For this review, take the finished solid that the model builds, in its own axes (mm). Face numbers are marked on the shaded views. A direction names the side the tool comes from. Give positions to 0.01 mm unless a question says otherwise; leave off trailing zeros. Write each loop counter-clockwise with the first axis right and the second up, starting at its lowest first coordinate (ties: lowest second). Pieces come first, ordered by that corner, then holes. Notation, with made-up numbers: (-19, 18) -> (16, 18) arc R34 ccw to (16, 48) -> close; hole circle Ø7 at (-17.75, 16.5). An arc over 180 degrees is marked (long way). Write item = value, one per line.
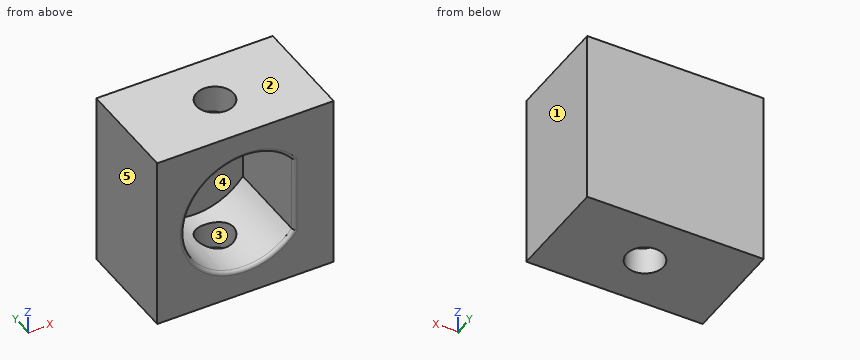
```python
from build123d import *

# Parameters (mm, degrees)
F0_W     = 50
F0_H     = 50
F1_DEPTH = 30
F3_R     = 1
F4_W     = 50
F4_H     = 50
F5_DEPTH = 5
F6_D     = 10.5


with BuildPart() as f1:
    # F0 (on Front) → F1 (new body)
    with BuildSketch(Plane.XZ):
        Rectangle(F0_W, F0_H)
        with BuildLine():
            ThreePointArc((13.65, -10.8710625056), (-17.45, 0), (13.65, 10.8710625056))
            Line((13.65, 10.8710625056), (13.65, -10.8710625056))
        make_face(mode=Mode.SUBTRACT)
    extrude(amount=F1_DEPTH)

    # F3
    f3_edges = [f1.edges().sort_by_distance(p)[0] for p in [
        (13.65, -30, 0),
        (-17.45, -30, 0),
    ]]
    fillet(f3_edges, radius=F3_R)

    # F4 (on face) → F5 (join)
    with BuildSketch(Plane.XZ):
        Rectangle(F4_W, F4_H)
    extrude(amount=F5_DEPTH)

    # F6 (through all)
    with Locations(Plane(origin=(0, 0, -25), x_dir=(1, 0, 0), z_dir=(0, 0, -1))):
        with Locations((0, 15)):
            Hole(F6_D / 2)


solid = f1.part
```
(1) Take a section at A-A (y = -15). Write out the cut boundary in (x, z), plus the area to 3 significant figures.
Answers below:
outline = (-25, -25) -> (-5.25, -25) -> (-5.25, -16.64) arc R17.45 cw to (-5.25, 16.64) -> (-5.25, 25) -> (-25, 25) -> close; (5.25, -25) -> (25, -25) -> (25, 25) -> (5.25, 25) -> (5.25, 16.64) arc R17.45 cw to (13.65, 10.87) -> (13.65, -10.87) arc R17.45 cw to (5.25, -16.64) -> close
area = 1,440 mm^2
(2) Take a section at D-D (y = -24). Write out the cut boundary in (x, z), plus the area to 3 significant figures.
Answers below:
outline = (-25, -25) -> (25, -25) -> (25, 25) -> (-25, 25) -> close; hole (13.65, -10.87) -> (13.65, 10.87) arc R17.45 ccw (long way) to start
area = 1,600 mm^2
(3) Take a section at B-B (z = 0). Write out the cut boundary in (x, y), plus the area to 3 significant figures.
Answers below:
outline = (-25, -30) -> (-18.45, -30) arc R1 ccw to (-17.45, -29) -> (-17.45, -5) -> (13.65, -5) -> (13.65, -29) arc R1 ccw to (14.65, -30) -> (25, -30) -> (25, 0) -> (-25, 0) -> close
area = 722 mm^2
(4) To check wall thickness, follow probe 1 along Z at (x, y) = (0, -22); probe 2 along X at (y, z) = (-7, -0.5); probe 3 along X at (y, z) = (-16, 5.5). State the ranges of each line that lie inside material, in increasing order.
Answers below:
probe_1 = -25 to -17.45, 17.45 to 25
probe_2 = -25 to -17.44, 13.65 to 25
probe_3 = -25 to -16.56, 13.65 to 25
(5) Tool access review of the marked faces 4 and 5: name each direction out of +Z, -Z, +X, -X, +Y, -Y from which nothing blocks a thin tool from reaching the whole face with its end or side.
Answers below:
face_4 = -Y
face_5 = +Z, -Z, -X, +Y, -Y
(6) Take a section at C-C (x = 0). Count the separate pieces of the cut face and the enclosed holes in it, plus the area to 3 significant figures.
Answers below:
separate_pieces = 3
enclosed_holes = 0
area = 469 mm^2
(7) For pin 1 (8.5 mm diameter, centred on x = 0, y = -15, fed in from +Z); pin 2 (9.5 mm diameter, centred on x = -9, z = 5.5, fed in from -Y), all flat-tipped, find the tip position at first contact; note any pin that passes through.
Answers below:
pin_1 = through
pin_2 = -5
(8) The part is to be moulded in two halves that separate along X. For the marked faces 1, 2 and 3, say which applies: released by +X, released by -X, zero draft, split by the parting line, or undercut.
Answers below:
face_1 = released by +X
face_2 = zero draft
face_3 = undercut
